from build123d import *

# Parameters (mm, degrees)
F10_R = 5
F11_R = 5
F12_R = 5


with BuildPart() as f2:
    # F2: sweep along a path in F1
    with BuildLine(Plane.XZ) as f2_path:
        Line((40, 0), (0, 0))
        Line((0, 0), (0, 120))
        Line((0, 120), (40, 120))
    # F0 (on Top) → F2 (sweep)
    with BuildSketch(Plane.XY):
        Polygon((-2, 13.2655382454), (0, 13.2655382454), (0, 18.2655382454), (2.5, 18.2655382454), (2.5, 13.2655382454), (4.5, 13.2655382454), (4.5, 20.2655382454), (-2, 20.2655382454), align=None)
    sweep(path=f2_path.line, transition=Transition.RIGHT)

    # F8: sweep along a path in F3
    with BuildLine(Plane.XZ) as f8_path:
        Line((0, 10), (0, 20))
    # F6 (on plane+point) → F8 (sweep)
    with BuildSketch(Plane.XY.offset(10)):
        with BuildLine():
            ThreePointArc((0, -2.5), (1.25, -1.25), (0, 0))
            Line((0, 0), (0, 13.2655382454))
            Line((0, 13.2655382454), (-2, 13.2655382454))
            Line((-2, 13.2655382454), (-2, -2.5))
            Line((-2, -2.5), (0, -2.5))
        make_face()
        with BuildLine():
            Line((4.5, 13.2655382454), (2.5, 13.2655382454))
            Line((2.5, 13.2655382454), (2.5, 4.5))
            ThreePointArc((2.5, 4.5), (1.25, 3.25), (2.5, 2))
            Line((2.5, 2), (4.5, 2))
            Line((4.5, 2), (4.5, 13.2655382454))
        make_face()
    sweep(path=f8_path.line)

    # F9: sweep along a path in F3
    with BuildLine(Plane.XZ) as f9_path:
        Line((0, 110), (0, 100))
    # F7 (on plane+point) → F9 (sweep)
    with BuildSketch(Plane.XY.offset(100)):
        with BuildLine():
            ThreePointArc((0, -2.5), (1.25, -1.25), (0, 0))
            Line((0, 0), (0, 13.2655382454))
            Line((0, 13.2655382454), (-2, 13.2655382454))
            Line((-2, 13.2655382454), (-2, -2.5))
            Line((-2, -2.5), (0, -2.5))
        make_face()
        with BuildLine():
            Line((4.5, 13.2655382454), (2.5, 13.2655382454))
            Line((2.5, 13.2655382454), (2.5, 4.5))
            ThreePointArc((2.5, 4.5), (1.25, 3.25), (2.5, 2))
            Line((2.5, 2), (4.5, 2))
            Line((4.5, 2), (4.5, 13.2655382454))
        make_face()
    sweep(path=f9_path.line)

    # F10
    f10_edges = [f2.edges().sort_by_distance(p)[0] for p in [
        (-1, 13.265538, 10),
        (3.5, 13.265538, 10),
        (-1, 13.265538, 20),
        (3.5, 13.265538, 20),
        (-1, 13.265538, 100),
        (3.5, 13.265538, 100),
        (3.5, 13.265538, 110),
        (-1, 13.265538, 110),
    ]]
    fillet(f10_edges, radius=F10_R)

    # F11
    f11_edges = [f2.edges().sort_by_distance(p)[0] for p in [
        (2.5, 15.765538, 117.5),
        (4.5, 16.765538, 115.5),
        (4.5, 16.765538, 4.5),
        (2.5, 15.765538, 2.5),
    ]]
    fillet(f11_edges, radius=F11_R)

    # F12
    f12_edges = [f2.edges().sort_by_distance(p)[0] for p in [
        (40, 13.265538, -1),
        (40, 13.265538, 3.5),
        (40, 13.265538, 121),
        (40, 13.265538, 116.5),
    ]]
    fillet(f12_edges, radius=F12_R)


solid = f2.part
For this review, take the finished solid that the model builds, in its own axes (mm). A direction names the side the tool comes from. Coordinates: 2 decimals unless noted, no trailing zeros. Write each loop counter-clockwise with the first axis right and the second up, starting at its lowest first coordinate (ties: lowest second). Pieces come first, ordered by that corner, then holes. Notation, with made-up numbers: (36, 8) -> (64, 8) arc R30 cw to (64, 38) -> close; hole circle Ø10 at (-23.5, 55.5). An arc over 180 degrees is marked (long way). Write each question's results on one line, items separated by ' | '. Start each with the question number.
1) Consider section D-D (z = 16.5). Write out the cut boundary in (x, y), plus the area to 3 significant figures.
2) Insertion check: pin 1 (1 mm diameter, centred on x = 3, y = 4.5, fed in from +Z); pin 2 (9 mm diameter, centred on y = 9, z = 53, fed in from +X); pin 3 (5 mm diameter, centred on y = 6, z = 21.5, fed in from -X); pin 4 (1.6 mm diameter, centred on x = 2.5, y = 5, fed in from -Z). Each pin has a flat end and moves straight along its axis. Give the tip position at first contact, or say it passes through.
3) Wall thickness on L1, parallel to Z at x = 22.5, y = 16.25; L2, parallel to X at y = 15.5, z = 80.5; L3, parallel to Z at x = 0.5, y = 16.5: over which ranges is each line inside the solid? List them lowest first. Write a range as [from, to].
4) Consider section A-A (y = 3.25). Write out the cut boundary in (x, z), plus the area to 3 significant figures.
5) Consider section C-C (z = 53.5). Write out the cut boundary in (x, y).
6) The part is to be moulded in two halves that separate along Z. For faces 4 (the face through (-1, 3, 110)), 5 (the face through (3, 2, 15)), 6 (the face through (6, 16.52, 114.07)), say which applies: +Z half, -Z half, draft (parallel to the pull), parting line (faces both ways), or undercut.
7) Consider section B-B (x = 33). Write out the cut boundary in (y, z).
8) For faces 1 (the face through (1.25, 3.22, 104.93)), 2 (the face through (-1, 3, 10)), 3 (the face through (2, 18.266, 46)), list the 3-axis set-ups (+Z, -Z, +X, -X, +Y, -Y) from which the entire face can be reached by the end or side of a thin tool; tool diameter is ignored.
Geometry says:
1) outline: (-2, -2.5) -> (0, -2.5) arc R1.25 ccw to (0, 0) -> (0, 18.27) -> (2.5, 18.27) -> (2.5, 4.5) arc R1.25 ccw to (2.5, 2) -> (4.5, 2) -> (4.5, 20.27) -> (-2, 20.27) -> close | area: 92.0 mm^2
2) pin 1: z = 110 | pin 2: x = 4.5 | pin 3: x = -2 | pin 4: z = 10
3) L1: [-2, 0], [2.5, 4.5], [115.5, 117.5], [120, 122] | L2: [-2, 0], [2.5, 4.5] | L3: [-2, 0], [120, 122]
4) outline: (-2, 10) -> (0, 10) -> (0, 20) -> (-2, 20) -> close; (-2, 100) -> (0, 100) -> (0, 110) -> (-2, 110) -> close; (1.25, 10) -> (4.5, 10) -> (4.5, 20) -> (1.25, 20) -> close; (1.25, 100) -> (4.5, 100) -> (4.5, 110) -> (1.25, 110) -> close | area: 105 mm^2
5) outline: (-2, 13.27) -> (0, 13.27) -> (0, 18.27) -> (2.5, 18.27) -> (2.5, 13.27) -> (4.5, 13.27) -> (4.5, 20.27) -> (-2, 20.27) -> close
6) face 4: +Z half | face 5: draft | face 6: undercut
7) outline: (13.27, -2) -> (20.27, -2) -> (20.27, 4.5) -> (13.27, 4.5) -> (13.27, 2.5) -> (18.27, 2.5) -> (18.27, 0) -> (13.27, 0) -> close; (13.27, 115.5) -> (20.27, 115.5) -> (20.27, 122) -> (13.27, 122) -> (13.27, 120) -> (18.27, 120) -> (18.27, 117.5) -> (13.27, 117.5) -> close
8) face 1: +Z, -Z | face 2: -Z, +X, -X, -Y | face 3: none
